Read the model definition and answer for the solid it produces. Units are mm, in the model's axes. Face numbers are marked on the shaded views. A direction names the side the tool comes from. Round coordinates to 2 decimals unless told otherwise and drop trailing zeros. Write each loop counter-clockwise with the first axis right and the second up, starting at its lowest first coordinate (ties: lowest second). Pieces come first, ordered by that corner, then holes.
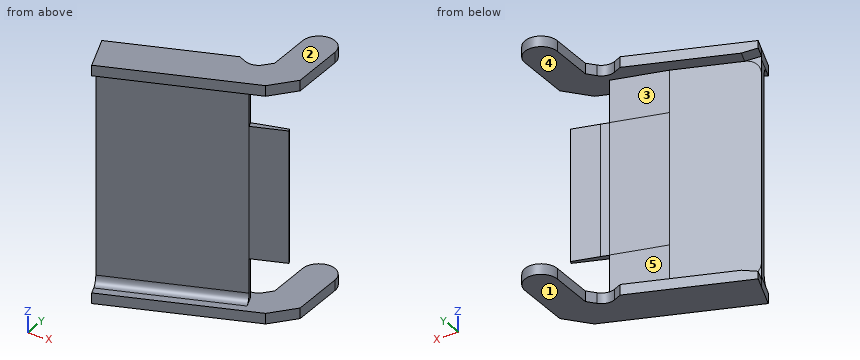
from build123d import *
from OCP.BRepFilletAPI import BRepFilletAPI_MakeChamfer

# Parameters (mm, degrees)
ESTRUSIONE_ESTRUSIONE1_DEPTH = 4
ESTRUSIONE_ESTRUSIONE2_DEPTH = 82
ESTRUSIONE_ESTRUSIONE3_START = 4
ESTRUSIONE_ESTRUSIONE3_DEPTH = 4
SCHIZZO6_W                   = 50
SCHIZZO6_H                   = 4
ESTRUSIONE_ESTRUSIONE4_DEPTH = 5
SMUSSO1_SIZE                 = 5.5
SMUSSO1_SIZE2                = 1.169061089
RACCORDO1_R                  = 3
SMUSSO2_SIZE                 = 5
RACCORDO2_START              = -86
RACCORDO2_DEPTH              = 4
RACCORDO2_2_DEPTH            = 4
SCHIZZO7_W                   = 50
SCHIZZO7_H                   = 2.5
ESTRUSIONE_ESTRUSIONE5_DEPTH = 13
SMUSSO3_SIZE                 = 20
SMUSSO3_SIZE_2               = 1.048155586
SMUSSO4_SIZE                 = 20
SMUSSO4_SIZE2                = 1.749773271
SMUSSO5_SIZE                 = 10
SMUSSO5_SIZE2                = 0.350328071


with BuildPart() as part:
    # Schizzo1 → Estrusione-Estrusione1 (new body)
    with BuildSketch(Plane.XY):
        with BuildLine():
            Line((4.891723927, 5.829729564), (4.891723927, 21.912236928))
            ThreePointArc((4.891723927, 21.912236928), (11.08058435, 28.101097351), (17.269444773, 21.912236928))
            Line((17.269444773, 21.912236928), (17.269444773, 1.912236928))
            Line((17.269444773, 1.912236928), (9.899185428, -6.871296125))
            Line((9.899185428, -6.871296125), (-42.94312967, -27.493410377))
            Line((-42.94312967, -27.493410377), (-46.57866514, -18.177677349))
            Line((-46.57866514, -18.177677349), (0, 0))
            Line((0, 0), (4.891723927, 5.829729564))
        make_face()
    extrude(amount=ESTRUSIONE_ESTRUSIONE1_DEPTH)

    # Schizzo4 → Estrusione-Estrusione2 (add)
    with BuildSketch(Plane.XY):
        Polygon((-45.124450952, -21.90397056), (1.454214188, -3.726293211), (0, 0), (-46.57866514, -18.177677349), align=None)
    extrude(amount=-ESTRUSIONE_ESTRUSIONE2_DEPTH)

    # Schizzo5 → Estrusione-Estrusione3 (add)
    with BuildSketch(Plane(origin=(0, 0, -82), x_dir=(-1, 0, 0), z_dir=(0, 0, -1)).offset(ESTRUSIONE_ESTRUSIONE3_START)):
        with BuildLine():
            Line((42.94312967, -27.493410377), (46.57866514, -18.177677349))
            Line((46.57866514, -18.177677349), (0, 0))
            Line((0, 0), (-4.891723927, 5.829729564))
            Line((-4.891723927, 5.829729564), (-4.891723927, 21.912236928))
            ThreePointArc((-4.891723927, 21.912236928), (-11.08058435, 28.101097351), (-17.269444773, 21.912236928))
            Line((-17.269444773, 21.912236928), (-17.269444773, 1.912236928))
            Line((-17.269444773, 1.912236928), (-9.899185428, -6.871296125))
            Line((-9.899185428, -6.871296125), (42.94312967, -27.493410377))
        make_face()
    extrude(amount=-ESTRUSIONE_ESTRUSIONE3_DEPTH)

    # Schizzo6 → Estrusione-Estrusione4 (add)
    with BuildSketch(Plane(origin=(0, 0, 0), x_dir=(0.9315733027957475, 0.36355354697516373, 0), z_dir=(-0.36355354697516373, 0.9315733027957475, 0))):
        with Locations((-25, 84)):
            Rectangle(SCHIZZO6_W, SCHIZZO6_H)
        with Locations((-25, -2)):
            Rectangle(SCHIZZO6_W, SCHIZZO6_H)
    extrude(amount=ESTRUSIONE_ESTRUSIONE4_DEPTH)

    # Smusso1: one chamfer whose edges measure the first distance from different faces: ONE call of the kernel's chamfer builder (chamfer() names one face for all edges)
    smusso1_edges_1 = [part.edges().sort_by_distance(p)[0] for p in [
        (-47.487549007, -15.848744092, -82),
    ]]
    smusso1_side_1 = [part.faces().sort_by_distance(p)[0] for p in [
        (-24.198216437, -6.759905417, -82),
    ]]
    smusso1_edges_2 = [part.edges().sort_by_distance(p)[0] for p in [
        (-47.487549007, -15.848744092, 0),
    ]]
    smusso1_side_2 = [part.faces().sort_by_distance(p)[0] for p in [
        (-24.198216437, -6.759905417, 0),
    ]]
    smusso1 = BRepFilletAPI_MakeChamfer(part.part.solid().wrapped)
    for e in smusso1_edges_1:
        smusso1.Add(SMUSSO1_SIZE, SMUSSO1_SIZE2, e.wrapped, smusso1_side_1[0].wrapped)  # the first distance lies on this face
    for e in smusso1_edges_2:
        smusso1.Add(SMUSSO1_SIZE, SMUSSO1_SIZE2, e.wrapped, smusso1_side_2[0].wrapped)  # the first distance lies on this face
    add(Compound.cast(smusso1.Shape()), mode=Mode.REPLACE)

    # Raccordo1
    raccordo1_edges = [part.edges().sort_by_distance(p)[0] for p in [
        (-21.835118382, -12.815131886, -82),
        (-21.835118382, -12.815131886, 0),
    ]]
    fillet(raccordo1_edges, radius=RACCORDO1_R)

    # Smusso2
    smusso2_edges = [part.edges().sort_by_distance(p)[0] for p in [
        (-1.817767735, 4.657866514, 2),
        (-1.817767735, 4.657866514, -84),
    ]]
    chamfer(smusso2_edges, length=SMUSSO2_SIZE - 0.0001)  # a hair under: the kernel refuses the full size

    # Raccordo2: read off the stored shape, not the designer's step
    # Raccordo2 outline → Raccordo2 (add)
    with BuildSketch(Plane.XY.offset(RACCORDO2_START)):
        with BuildLine():
            Line((0, 0), (2.407895765, 2.869618428))
            ThreePointArc((2.407895765, 2.869618428), (-0.284030607, 1.214852073), (-3.430579557, 1.504591587))
            Line((-3.430579557, 1.504591587), (0, 0))
        make_face()
    extrude(amount=RACCORDO2_DEPTH)

    # Raccordo2 2 outline → Raccordo2 2 (add)
    with BuildSketch(Plane.XY):
        with BuildLine():
            Line((0, 0), (2.407895765, 2.869618428))
            ThreePointArc((2.407895765, 2.869618428), (-0.284030607, 1.214852073), (-3.430579557, 1.504591587))
            Line((-3.430579557, 1.504591587), (0, 0))
        make_face()
    extrude(amount=RACCORDO2_2_DEPTH)

    # Schizzo7 → Estrusione-Estrusione5 (add)
    with BuildSketch(Plane(origin=(0, 0, 0), x_dir=(0, 0, -1), z_dir=(0.9315733027957472, 0.3635535469751644, 0))):
        with Locations((41, -2.75)):
            Rectangle(SCHIZZO7_W, SCHIZZO7_H)
    extrude(amount=ESTRUSIONE_ESTRUSIONE5_DEPTH)

    # Smusso3
    # the kernel refuses this chamfer: 20, 1.048155586 mm, written as the material it takes off along each edge
    with BuildSketch(Plane(origin=(12.655783257, 3.328836156, -16), x_dir=(-0.9315733027957472, -0.3635535469751644, 0), z_dir=(0, 0, -1))) as smusso3_piece_1_section:
        Polygon((SMUSSO3_SIZE, 0), (0, -SMUSSO3_SIZE_2), (0, 0), align=None)
    smusso3_piece_1 = extrude(amount=50, mode=Mode.PRIVATE)
    smusso3_piece_1 = split(smusso3_piece_1, bisect_by=Plane(origin=(0.54533032, -1.397359954, -16), z_dir=(0.9315733027957472, 0.36355354697516445, 0)), keep=Keep.TOP, mode=Mode.PRIVATE)
    add(smusso3_piece_1, mode=Mode.SUBTRACT)

    # Smusso4
    smusso4_edges = [part.edges().sort_by_distance(p)[0] for p in [
        (0, 0, -41),
    ]]
    smusso4_side = [part.faces().sort_by_distance(p)[0] for p in [
        (-23.323124739, -9.102026325, -41),
    ]]
    chamfer(smusso4_edges, length=SMUSSO4_SIZE, length2=SMUSSO4_SIZE2, reference=smusso4_side[0])

    # Smusso5
    smusso5_edges = [part.edges().sort_by_distance(p)[0] for p in [
        (13.036843938, 2.352402395, -41),
    ]]
    smusso5_side = [part.faces().sort_by_distance(p)[0] for p in [
        (6.857772748, 0.306645312, -41),
    ]]
    chamfer(smusso5_edges, length=SMUSSO5_SIZE, length2=SMUSSO5_SIZE2, reference=smusso5_side[0])


solid = part.part
Q1. Flat-ended cylindrical pins translate along their axes: pin 1 Ø8 at (x, z) = (-4.5, -69) entering from -Y; pin 2 Ø6 at (x, z) = (-39.5, -45.5) entering from +Y; pin 3 Ø6 at (x, z) = (-6.5, -37.5) entering from +Y. Find the tip coordinate at first contact, or state that the pin passes through.
Verdict:
pin 1: stops at y = -7.61
pin 2: stops at y = -14.24
pin 3: stops at y = -2.84
Q2. Section D-D (y = 23.5) is taken. Determine the outline of the cut face in (x, z), then the cut area to 3 significant figures.
Verdict:
outline: (5.1, -86) - (17.06, -86) - (17.06, -82) - (5.1, -82) - close; (5.1, 0) - (17.06, 0) - (17.06, 4) - (5.1, 4) - close
area: 95.7 mm2
Q3. Determine the mould class of the marked faces 1, 2 and 3 for opening direction Z: pulls with the +Z half, pulls with the -Z half, needs draft (parallel to the pull), parting line crosses it, or undercut.
Verdict:
face 1: pulls with the -Z half
face 2: pulls with the +Z half
face 3: undercut
Q4. Section A-A (y = 12) is taken. Determine the outline of the cut face in (x, z).
Verdict:
outline: (4.89, -86) - (17.27, -86) - (17.27, -82) - (4.89, -82) - close; (4.89, 0) - (17.27, 0) - (17.27, 4) - (4.89, 4) - close
Q5. Section B-B (x = 11.5) is taken. Determine the outline of the cut face in (y, z), then the cut area to 3 significant figures.
Verdict:
outline: (-4.96, -86) - (28.09, -86) - (28.09, -82) - (-4.96, -82) - close; (-4.96, 0) - (28.09, 0) - (28.09, 4) - (-4.96, 4) - close; (0.19, -66) - (1.54, -66) - (1.54, -16) - (0.19, -16) - close
area: 332 mm2
Q6. Section C-C (z = -9) is taken. Determine the outline of the cut face in (x, y).
Verdict:
outline: (-46.58, -18.18) - (-45.12, -21.9) - (1.45, -3.73) - (0.64, -1.63) - (-18.63, -7.27) - close
Q7. Straight lines are drawn through the part: probe 1 along Z at (x, y) = (-2, -8); probe 2 along Y at (x, z) = (-42, -45.5); probe 3 along Y at (x, z) = (-35, -57.5). For each, find the intervals that lie inside material, in ascending order.
Verdict:
probe 1: z = -86 to -81.99, -0.01 to 4
probe 2: y = -20.68 to -16.39
probe 3: y = -17.95 to -13.66
Q8. Which of the six approach directions +Z, -Z, +X, -X, +Y, -Y give full straight-line access (tool end or side, diameter ignored) to the marked faces 4 and 5?
Verdict:
face 4: none
face 5: -X, +Y
